```python
from build123d import *

# Parameters (mm, degrees)
BOSS_EXTRUDE1_DEPTH = 25
SKETCH2_W           = 10
SKETCH2_H           = 64.104672306
BOSS_EXTRUDE2_DEPTH = 60
CUT_EXTRUDE1_DEPTH  = 60
SKETCH4_R           = 1.5
CUT_EXTRUDE2_DEPTH  = 60
FILLET1_R           = 2
SKETCH13_R          = 1.5
CUT_EXTRUDE3_DEPTH  = 10


with BuildPart() as part:
    # Sketch1 → Boss-Extrude1 (new, symmetric)
    with BuildSketch(Plane.XY):
        Polygon((0, 76.71875), (-10, 76.71875), (-10, -223.28125), (60, -223.28125), (60, -213.28125), (0, -213.28125), align=None)
    extrude(amount=BOSS_EXTRUDE1_DEPTH, both=True)

    # Sketch2 → Boss-Extrude2 (add)
    with BuildSketch(Plane(origin=(0, 0, 0), x_dir=(0, 0, -1), z_dir=(1, 0, 0))):
        with Locations((0, -181.228913847)):
            Rectangle(SKETCH2_W, SKETCH2_H)
    extrude(amount=BOSS_EXTRUDE2_DEPTH)

    # Sketch3 → Cut-Extrude1 (cut)
    with BuildSketch(Plane.XY.offset(5)):
        Polygon((0, -149.176577694), (60, -213.28125), (60, -149.176577694), align=None)
    extrude(amount=-CUT_EXTRUDE1_DEPTH, mode=Mode.SUBTRACT)

    # Sketch4 → Cut-Extrude2 (cut)
    with BuildSketch(Plane(origin=(0, -213.28125, 0), x_dir=(1, 0, 0), z_dir=(0, 1, 0))):
        with Locations(Location((15, 15, 0), (0, 0, 270))):
            Circle(SKETCH4_R)
        with Locations(Location((15, -15, 0), (0, 0, 270))):
            Circle(SKETCH4_R)
        with Locations(Location((45, -15, 0), (0, 0, 270))):
            Circle(SKETCH4_R)
        with Locations(Location((45, 15, 0), (0, 0, 270))):
            Circle(SKETCH4_R)
    extrude(amount=-CUT_EXTRUDE2_DEPTH, mode=Mode.SUBTRACT)

    # Fillet1
    fillet1_edges = [part.edges().sort_by_distance(p)[0] for p in [
        (0, -181.228913847, 5),
        (30, -213.28125, 5),
        (0, -181.228913847, -5),
        (30, -213.28125, -5),
        (0, -149.176577694, 0),
    ]]
    fillet(fillet1_edges, radius=FILLET1_R)

    # Sketch13 → Cut-Extrude3 (cut)
    with BuildSketch(Plane(origin=(0, 0, 0), x_dir=(0, 0, -1), z_dir=(1, 0, 0))):
        with Locations(Location((0, 26.71875, 0), (0, 0, 90))):
            Circle(SKETCH13_R)
        with Locations(Location((0, -23.28125, 0), (0, 0, 90))):
            Circle(SKETCH13_R)
    extrude(amount=-CUT_EXTRUDE3_DEPTH, mode=Mode.SUBTRACT)


solid = part.part
```
Source: CAD feature listing. Evaluate the final solid. Frame: model axes, mm. A direction names the side the tool comes from. Coordinates: 2 decimals unless noted, no trailing zeros. Write each loop counter-clockwise with the first axis right and the second up, starting at its lowest first coordinate (ties: lowest second). Pieces come first, ordered by that corner, then holes. Notation, with made-up numbers: (62, 89.25) -> (95, 89.25) arc R17 cw to (95, 101.25) -> close; hole circle Ø8 at (58, 47). An arc over 180 degrees is marked (long way). Return JSON: item names as keys, results as strings. Group by question number.
1) Contact query for flat-ended pins moving along their axis: P1, Ø12, axis at x = 47, z = 4, coming from the +Y side; P2, Ø17, axis at x = 43, y = -178.5, coming from the -Z side; P3, Ø5, axis at y = 26.72, z = 0, coming from the -X side; P4, Ø9, axis at x = 32.5, z = 15, coming from the +Y side. Output: stop coordinate, or through.
2) Section query D-D, the plane y = -39.5. Return loops of the section in (x, z).
3) Section query A-A, the plane y = -166.5. Return loops of the section in (x, z), plus the area to 3 significant figures.
4) Section query B-B, the plane z = 21.5. Return loops of the section in (x, y).
5) Section query C-C, the plane x = 21. Return loops of the section in (y, z), plus the area to 3 significant figures.
6) Set-up query: faces 1 (the face through (30, -213.281, -16)), 2 (the face through (60, -218, 0)), 3 (the face through (30, -213.281, 16)). Return all of +Z, -Z, +X, -X, +Y, -Y with unobstructed straight access to the full face (end or side cutting, diameter ignored); none if empty.
7) Ray query, line 1 along X through (y, z) = (-220, -15); line 2 along Y through (x, z) = (55.5, -20.5); line 3 along X through (y, z) = (-26, -1). Return the intervals inside material, ascending.
From the geometry:
{
 "1": {"P1": "y = -192.98", "P2": "through", "P3": "x = -10", "P4": "y = -213.28"},
 "2": {"outline": "(-10, -25) -> (0, -25) -> (0, 25) -> (-10, 25) -> close"},
 "3": {"outline": "(-10, -25) -> (0, -25) -> (0, -7) arc R2 cw to (2, -5) -> (16.21, -5) -> (16.21, 5) -> (2, 5) arc R2 cw to (0, 7) -> (0, 25) -> (-10, 25) -> close", "area": "664 mm²"},
 "4": {"outline": "(-10, -223.28) -> (60, -223.28) -> (60, -213.28) -> (0, -213.28) -> (0, 76.72) -> (-10, 76.72) -> close"},
 "5": {"outline": "(-223.28, -25) -> (-213.28, -25) -> (-213.28, -7) arc R2 cw to (-211.28, -5) -> (-171.61, -5) -> (-171.61, 5) -> (-211.28, 5) arc R2 cw to (-213.28, 7) -> (-213.28, 25) -> (-223.28, 25) -> close", "area": "918 mm²"},
 "6": {"face 1": "-Z, +X, +Y", "face 2": "+Z, -Z, +X, +Y, -Y", "face 3": "+Z, +X, +Y"},
 "7": {"line 1": "-10 to 13.5, 16.5 to 43.5, 46.5 to 60", "line 2": "-223.28 to -213.28", "line 3": "-10 to 0"}
}
